```python
from build123d import *

# Parameters (mm, degrees)
SKETCH1_W           = 55
SKETCH1_H           = 55
BOSS_EXTRUDE1_DEPTH = 5
CHAMFER1_SIZE       = 5
SKETCH2_R           = 1.95
SKETCH2_R_2         = 1.9
SKETCH2_R_3         = 10
CUT_EXTRUDE1_DEPTH  = 10
SKETCH3_R           = 17.5
CUT_EXTRUDE2_DEPTH  = 1.5


with BuildPart() as part:
    # Sketch1 → Boss-Extrude1 (new body)
    with BuildSketch(Plane.XY):
        Rectangle(SKETCH1_W, SKETCH1_H)
    extrude(amount=BOSS_EXTRUDE1_DEPTH)

    # Chamfer1
    chamfer1_edges = [part.edges().sort_by_distance(p)[0] for p in [
        (-27.5, -27.5, 2.5),
        (27.5, -27.5, 2.5),
        (27.5, 27.5, 2.5),
        (-27.5, 27.5, 2.5),
    ]]
    chamfer(chamfer1_edges, length=CHAMFER1_SIZE)

    # Sketch2 → Cut-Extrude1 (cut)
    with BuildSketch(Plane(origin=(0, 0, 0), x_dir=(-1, 0, 0), z_dir=(0, 0, -1))):
        with Locations((0, 14.5)):
            Circle(SKETCH2_R)
        with Locations((-22.5, 22.5)):
            Circle(SKETCH2_R_2)
        with Locations((22.5, 22.5)):
            Circle(SKETCH2_R_2)
        with Locations((22.5, -22.5)):
            Circle(SKETCH2_R_2)
        with Locations((-22.5, -22.5)):
            Circle(SKETCH2_R_2)
        Circle(SKETCH2_R_3)
        with Locations((0, -14.5)):
            Circle(SKETCH2_R)
    extrude(amount=-CUT_EXTRUDE1_DEPTH, mode=Mode.SUBTRACT)

    # Sketch3 → Cut-Extrude2 (cut)
    with BuildSketch(Plane(origin=(0, 0, 0), x_dir=(-1, 0, 0), z_dir=(0, 0, -1))):
        Circle(SKETCH3_R)
    extrude(amount=-CUT_EXTRUDE2_DEPTH, mode=Mode.SUBTRACT)


solid = part.part
```
Input: part model. Units: mm. Frame: model coordinates. A direction names the side the tool comes from. Give positions to 0.01 mm unless a question says otherwise; leave off trailing zeros. Order: outer loops, then holes, each group sorted by start corner. A loop starts at its lowest first (then second) coordinate and runs counter-clockwise, first axis right, second up.
1. Pin query (flat end, axial travel): pin 1 Ø17.5 at (x, y) = (-1.5, -5) entering from -Z. Return the tip coordinate at first contact, or that it passes through.
Computed:
pin 1: stops at z = 1.5
2. Set-up query: faces 4 (the face through (13.887, -10.648, 0.74)), 5 (the face through (-25, 25, 2)). Return all of +Z, -Z, +X, -X, +Y, -Y with unobstructed straight access to the full face (end or side cutting, diameter ignored); none if empty.
Computed:
face 4: -Z
face 5: +Z, -Z, -X, +Y
3. Line query: probe 1 along Y at (x, z) = (-21, 3.5); probe 2 along Y at (x, z) = (22.5, 2.45); probe 3 along X at (y, z) = (24, 2.1). Output: solid intervals per line, ascending.
Computed:
probe 1: y = -27.5 to -23.67, -21.33 to 21.33, 23.67 to 27.5
probe 2: y = -27.5 to -24.4, -20.6 to 20.6, 24.4 to 27.5
probe 3: x = -26 to -23.67, -21.33 to 21.33, 23.67 to 26
4. Cut plane C-C (y = 0). Return loops of the section in (x, z), and give its area (4 significant figures).
Computed:
outline: (-27.5, 0) - (-17.5, 0) - (-17.5, 1.5) - (-10, 1.5) - (-10, 5) - (-27.5, 5) - close; (10, 1.5) - (17.5, 1.5) - (17.5, 0) - (27.5, 0) - (27.5, 5) - (10, 5) - close
area: 152.5 mm2
5. Cut plane A-A (z = 3.7). Return loops of the section in (x, y).
Computed:
outline: (-27.5, -22.5) - (-22.5, -27.5) - (22.5, -27.5) - (27.5, -22.5) - (27.5, 22.5) - (22.5, 27.5) - (-22.5, 27.5) - (-27.5, 22.5) - close; hole circle Ø3.8 at (-22.5, -22.5); hole circle Ø3.8 at (-22.5, 22.5); hole circle Ø20 at (0, 0); hole circle Ø3.9 at (0, -14.5); hole circle Ø3.9 at (0, 14.5); hole circle Ø3.8 at (22.5, -22.5); hole circle Ø3.8 at (22.5, 22.5)
6. Cut plane B-B (x = 0). Return loops of the section in (y, z), and give its area (3 significant figures).
Computed:
outline: (-27.5, 0) - (-17.5, 0) - (-17.5, 1.5) - (-16.45, 1.5) - (-16.45, 5) - (-27.5, 5) - close; (-12.55, 1.5) - (-10, 1.5) - (-10, 5) - (-12.55, 5) - close; (10, 1.5) - (12.55, 1.5) - (12.55, 5) - (10, 5) - close; (16.45, 1.5) - (17.5, 1.5) - (17.5, 0) - (27.5, 0) - (27.5, 5) - (16.45, 5) - close
area: 125 mm2
7. Draft query along Y for faces 1 (the face through (0, 27.5, 2)), 2 (the face through (25, -25, 2)), 3 (the face through (-21.1, -21.216, 2.465)). Return one class per face: released by +Y, released by -Y, zero draft, split by the parting line, or undercut.
Computed:
face 1: released by +Y
face 2: released by -Y
face 3: undercut
8. Cut plane D-D (x = 8.5). Return loops of the section in (y, z).
Computed:
outline: (-27.5, 0) - (-15.3, 0) - (-15.3, 1.5) - (-5.27, 1.5) - (-5.27, 5) - (-27.5, 5) - close; (5.27, 1.5) - (15.3, 1.5) - (15.3, 0) - (27.5, 0) - (27.5, 5) - (5.27, 5) - close
